Design review of the part built by this model. Coordinates are the model's own, in mm. A direction names the side the tool comes from. Coordinates: 2 decimals unless noted, no trailing zeros. Loops run counter-clockwise (first coordinate to the right, second up) from the corner with the lowest first, then second, coordinate; pieces in that order, holes last. Notation, with made-up numbers: (71.25, 80) -> (96.25, 80) arc R33 ccw to (96.25, 117) -> close; hole circle Ø7 at (-0.5, 59.5). An arc over 180 degrees is marked (long way). One line per item, written item: value. Start each with the question number.
1. Draft analysis for pull direction X (two halves, no side actions). For faces 5 (the flat face through (0, 7, -1)), 6 (the flat face through (28.5, 0, 1)), 7 (the flat face through (-21.25, 0, -2)), 8 (the flat face through (6.5, 9, -1)), state which applies: pulls with the +X half, pulls with the -X half, needs draft (parallel to the pull), parting line crosses it, or undercut.
2. For probe 1 along Y at (x, z) = (3, -3.75); probe 2 along X at (y, z) = (-4.5, -1), list the stretches that pass through material, from the lowest coordinate up.
3. Add section A-A on z = -3. Write out the cut boundary in (x, y).
4. Machinability: for faces 1 (the flat face through (15, 10.5, -1)), 2 (the flat face through (21.25, 0, -2)), 3 (the flat face through (-6.5, 9, -1)), 4 (the flat face through (-25, 0, 0)), which of the approach directions +Z, -Z, +X, -X, +Y, -Y give a long, thin tool a straight path to every point of the face, cutting with its end or side? Answer none if there is none.
5. Insertion check: pin 1 (8 mm diameter, centred on x = -26, y = 4, fed in from -Z); pin 2 (1.8 mm diameter, centred on y = 8, z = -3, fed in from +X); pin 3 (4 mm diameter, centred on y = 5, z = -1.5, fed in from -X); pin 4 (4 mm diameter, centred on x = 0.5, z = -1.5, fed in from +Y). Each pin has a flat end and moves straight along its axis. Give the tip position at first contact, or say it passes through.
6. Add section B-B on y = -8.5. Write out the cut boundary in (x, z), plus the area to 3 significant figures.
7. Add section C-C on x = -24. Write out the cut boundary in (y, z), plus the area to 3 significant figures.
```python
from build123d import *

# Parameters (mm, degrees)
SKETCH1_W           = 57
SKETCH1_H           = 21
BOSS_EXTRUDE1_DEPTH = 2.5
SKETCH2_W           = 42.5
SKETCH2_H           = 21
BOSS_EXTRUDE2_DEPTH = 5
SKETCH3_W           = 13
SKETCH3_H           = 3.5
CUT_EXTRUDE1_DEPTH  = 8.5


with BuildPart() as part:
    # Sketch1 → Boss-Extrude1 (new body)
    with BuildSketch(Plane.XY):
        Rectangle(SKETCH1_W, SKETCH1_H)
    extrude(amount=BOSS_EXTRUDE1_DEPTH)

    # Sketch2 → Boss-Extrude2 (add)
    with BuildSketch(Plane(origin=(0, 0, 0), x_dir=(-1, 0, 0), z_dir=(0, 0, -1))):
        Rectangle(SKETCH2_W, SKETCH2_H)
    extrude(amount=BOSS_EXTRUDE2_DEPTH)

    # Sketch3 → Cut-Extrude1 (cut, through all)
    with BuildSketch(Plane.XY.offset(2.5)):
        with Locations((0, 8.75)):
            Rectangle(SKETCH3_W, SKETCH3_H)
    extrude(amount=-CUT_EXTRUDE1_DEPTH, mode=Mode.SUBTRACT)


solid = part.part
```
Worked answers:
1. face 5: undercut
1. face 6: pulls with the +X half
1. face 7: pulls with the -X half
1. face 8: undercut
2. probe 1: y = -10.5 to 7
2. probe 2: x = -21.25 to 21.25
3. outline: (-21.25, -10.5) -> (21.25, -10.5) -> (21.25, 10.5) -> (6.5, 10.5) -> (6.5, 7) -> (-6.5, 7) -> (-6.5, 10.5) -> (-21.25, 10.5) -> close
4. face 1: +Z, -Z, +X, -X, +Y
4. face 2: -Z, +X, +Y, -Y
4. face 3: +Z, -Z, +Y
4. face 4: -Z, -X, +Y, -Y
5. pin 1: stops at z = 0
5. pin 2: stops at x = 21.25
5. pin 3: stops at x = -28.5
5. pin 4: stops at y = 7
6. outline: (-28.5, 0) -> (-21.25, 0) -> (-21.25, -5) -> (21.25, -5) -> (21.25, 0) -> (28.5, 0) -> (28.5, 2.5) -> (-28.5, 2.5) -> close
6. area: 355 mm²
7. outline: (-10.5, 0) -> (10.5, 0) -> (10.5, 2.5) -> (-10.5, 2.5) -> close
7. area: 52.5 mm²
